Check sheet for the modelled part. Datum: model origin and axes. Units: mm. A direction names the side the tool comes from. Give positions to 0.01 mm unless a question says otherwise; leave off trailing zeros. Order: outer loops, then holes, each group sorted by start corner. A loop starts at its lowest first (then second) coordinate and runs counter-clockwise, first axis right, second up.
Item 1: Sectioned sample at C-C on y = 0. Record the boundary of the cut face in (x, z).
Item 2: Release check for a two-part mould opening along Y. For faces 3 (the cylindrical face through (-12.5, -0.1, 1.5)), 4 (the flat face through (0, 0, 1.6)), 5 (the cylindrical face through (17.986, -4.569, 0.811)) record: released by +Y, released by -Y, zero draft, split by the parting line, or undercut.
Item 3: Sectioned sample at A-A on x = 10. Record the boundary of the cut face in (y, z), and give its area (3 significant figures).
Item 4: Access from +Z, -Z, +X, -X, +Y, -Y to the whole of each face (thin tool, end or side, straight path). Record for faces 1 (the cylindrical face through (13.3, -1, 2.3)), 2 (the flat face through (0, 5, 1)).
Item 5: Gauge pin test, flat ends, axial feed: P1, Ø1.5, axis at x = 13.5, y = -3, coming from the +Z side; P2, Ø4.5, axis at x = 10, y = 0, coming from the +Z side; P3, Ø1, axis at x = 6.5, z = 2.5, coming from the +Y side. Record the tip position at first contact, or that the pin passes through.
Item 6: Sectioned sample at D-D on x = 1.5. Record the boundary of the cut face in (y, z).
Item 7: Sectioned sample at B-B on z = 2.3. Record the boundary of the cut face in (x, y).
Item 8: Material ranges on line 1 along X through (y, z) = (-2, 1.05); line 2 along X through (y, z) = (-0.75, 0.4); line 3 along X through (y, z) = (0.75, 2.35), recorded low to high.
Autodesk Inventor part; units mm, degrees
ref_plane "YZ Plane" through (0, 0, 0) normal (1, 0, 0) x (0, 1, 0)
ref_plane "XZ Plane" through (0, 0, 0) normal (0, 1, 0) x (-1, 0, 0)
ref_plane "XY Plane" through (0, 0, 0) normal (0, 0, 1) x (1, 0, 0)
sketch "Sketch1" plane through (0, 0, 0) normal (0, 0, 1) x (1, 0, 0)
  line L0 (-18.44, 5) -> (18.44, 5)
  line L1 (18.44, 5) -> (18.44, -5)
  line L2 (18.44, -5) -> (-18.44, -5)
  line L3 (-18.44, -5) -> (-18.44, 5)
  line L4 (0, 5) -> (0, -5) construction
  line L5 (-18.44, 0) -> (18.44, 0) construction
  circle A0 centre (-10, 0) radius 2.5
  circle A1 centre (10, 0) radius 2.5
  point P0 (0, 0)
  dimension "d0" = 10
  dimension "d1" = 36.88
  dimension "d2" = 5
  dimension "d3" = 20
extrude "Extrusion1" add sketch "Sketch1" along normal blind 1.6
sketch "Sketch2" plane through (0, 0, 1.6) normal (0, 0, 1) x (1, 0, 0)
  circle A0 centre (10, 0) radius 2.5
  circle A1 centre (-10, 0) radius 2.5
  circle A2 centre (-10, 0) radius 3.45
  circle A3 centre (10, 0) radius 3.45
  point P0 (0, 0)
  dimension "d6" = 6.9
  dimension "d7" = 6.9
extrude "Extrusion2" add sketch "Sketch2" along normal blind 1.4
thread "Thread1"
thread "Thread2"
fillet "Fillet1" radius 1.51 4 edges at (18.44, 5, 0.8) (18.44, -5, 0.8) (-18.44, -5, 0.8) (-18.44, 5, 0.8)
properties part number "doube t-nut"
Report:
1. outline: (-18.44, 0) - (-12.5, 0) - (-12.5, 3) - (-13.45, 3) - (-13.45, 1.6) - (-18.44, 1.6) - close; (-7.5, 0) - (7.5, 0) - (7.5, 3) - (6.55, 3) - (6.55, 1.6) - (-6.55, 1.6) - (-6.55, 3) - (-7.5, 3) - close; (12.5, 0) - (18.44, 0) - (18.44, 1.6) - (13.45, 1.6) - (13.45, 3) - (12.5, 3) - close
2. face 3: undercut
2. face 4: zero draft
2. face 5: released by -Y
3. outline: (-5, 0) - (-2.5, 0) - (-2.5, 3) - (-3.45, 3) - (-3.45, 1.6) - (-5, 1.6) - close; (2.5, 0) - (5, 0) - (5, 1.6) - (3.45, 1.6) - (3.45, 3) - (2.5, 3) - close
3. area: 10.7 mm2
4. face 1: +Z
4. face 2: +Z, -Z, +X, -X, +Y
5. P1: stops at z = 1.6
5. P2: passes through
5. P3: stops at y = 1.7
6. outline: (-5, 0) - (5, 0) - (5, 1.6) - (-5, 1.6) - close
7. outline: circle Ø6.9 at (-10, 0); circle Ø6.9 at (10, 0); hole circle Ø5 at (-10, 0); hole circle Ø5 at (10, 0)
8. line 1: x = -18.44 to -11.5, -8.5 to 8.5, 11.5 to 18.44
8. line 2: x = -18.44 to -12.38, -7.62 to 7.62, 12.38 to 18.44
8. line 3: x = -13.37 to -12.38, -7.62 to -6.63, 6.63 to 7.62, 12.38 to 13.37
